Answer from the drawing. Dimensions are ordinates in mm from the lowest x, y and z of the part. A direction names the side the tool comes from. Coordinates: 2 decimals unless noted, no trailing zeros. Write each loop counter-clockwise with the first axis right and the second up, starting at its lowest first coordinate (ties: lowest second). Pieces come first, ordered by that corner, then holes.
(1) Straight lines are drawn through the part: line 1 along Y through (x, z) = (6, 5.75); line 2 along X through (y, z) = (43, 6) (1 decimal); line 3 along X through (y, z) = (26.5, 9) (1 decimal). For each, find the intervals that lie inside material, in ascending order.
(2) The part is cut by section B-B, the plane z = 5.5. Determine the outline of the cut face in (x, y) (1 decimal).
(3) The part is cut by section C-C, the plane x = 7.75. Determine the outline of the cut face in (y, z) (1 decimal).
(4) Which of the six approach directions +Z, -Z, +X, -X, +Y, -Y give full straight-line access (tool end or side, diameter ignored) to the marked faces 1 and 2?
(5) The part is cut by section A-A, the plane y = 25.5. Determine the outline of the cut face in (x, z) (1 decimal), and give its area (3 significant figures).
(6) The part is cut by section D-D, the plane y = 47. Determine the outline of the cut face in (x, z) (1 decimal).
(7) Given pin 1 (1.5 mm diameter, centred on y = 34.5, z = 5.5, fed in from -X) (1 decimal); pin 2 (2.5 mm diameter, centred on y = 13, z = 1.5, fed in from +X) (1 decimal), each flat-ended and moving along its own axis, determine where each tip first touches the part or whether it passes through.
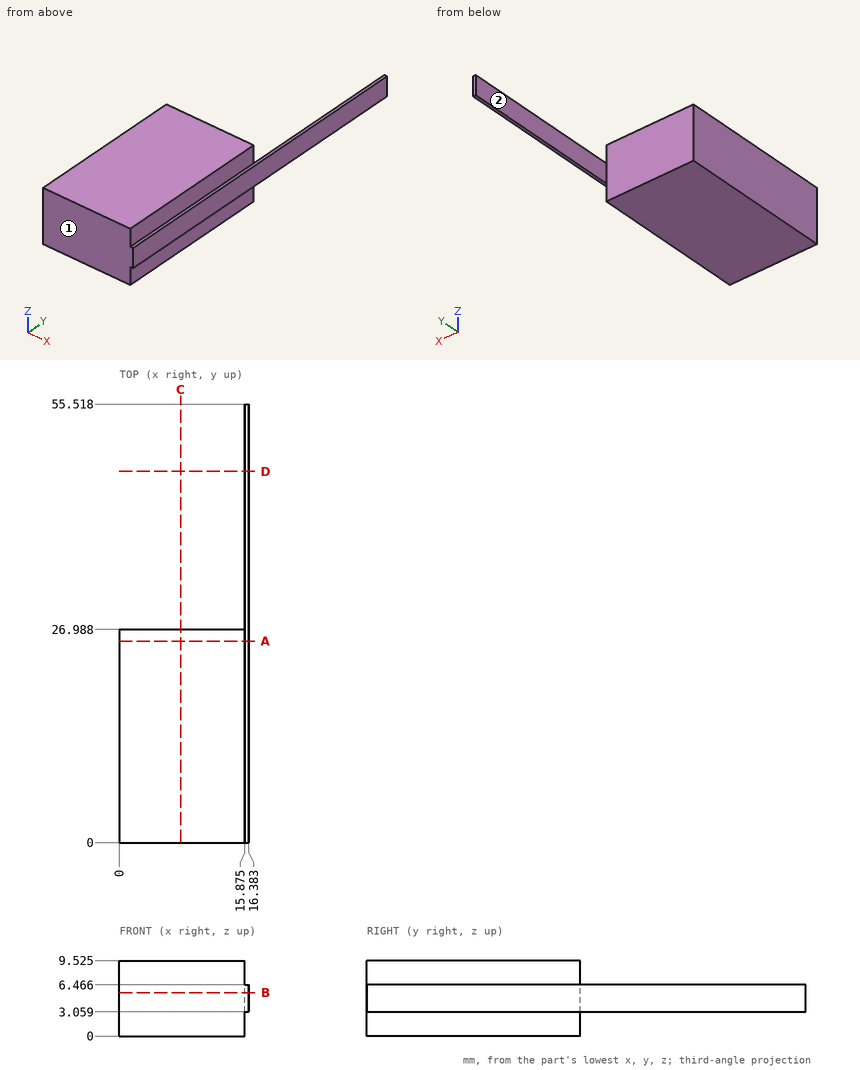
Computed:
1. line 1: y = 0 to 26.99
1. line 2: x = 15.9 to 16.4
1. line 3: x = 0 to 15.9
2. outline: (0, 0) - (16.4, 0) - (16.4, 55.5) - (15.9, 55.5) - (15.9, 27) - (0, 27) - close
3. outline: (0, 0) - (27, 0) - (27, 9.5) - (0, 9.5) - close
4. face 1: +Z, -Z, +X, -X, -Y
4. face 2: +Z, -Z, -X, +Y
5. outline: (0, 0) - (15.9, 0) - (15.9, 3.1) - (16.4, 3.1) - (16.4, 6.5) - (15.9, 6.5) - (15.9, 9.5) - (0, 9.5) - close
5. area: 153 mm2
6. outline: (15.9, 3.1) - (16.4, 3.1) - (16.4, 6.5) - (15.9, 6.5) - close
7. pin 1: stops at x = 15.9
7. pin 2: stops at x = 15.9
